Read the model definition and answer for the solid it produces. Units are mm, in the model's axes. Give positions to 0.01 mm unless a question says otherwise; leave off trailing zeros. Loops run counter-clockwise (first coordinate to the right, second up) from the corner with the lowest first, then second, coordinate; pieces in that order, holes last. Notation, with made-up numbers: (-27.75, 58) - (18.25, 58) arc R24 ccw to (18.25, 70) - close; hole circle Ø10 at (86, 20). An arc over 180 degrees is marked (long way). Put each result on its own line as item: value. Start each with the question number.
1. Given pin 1 Ø12 at (x, y) = (115.5, 28) entering from +Z; pin 2 Ø10 at (x, z) = (-159, 6.5) entering from +Y; pin 3 Ø6 at (x, y) = (-97, 34.5) entering from +Z; pin 4 Ø4.5 at (x, y) = (-194.5, -25) entering from -Z, each flat-ended and moving along its own axis, determine where each tip first touches the part or whether it passes through.
2. A cutting plane is placed at B-B, the plane y = 25.5. Determine the outline of the cut face in (x, z), plus the area to 3 significant figures.
3. Consider L1, parallel to Y at x = -422, z = 1.75; L2, parallel to Y at x = 131, z = 2.25; L3, parallel to Y at x = 32.5, z = 7.75. Determine where each line is inside the solid, lowest interval first. Write a range as from..to.
```python
from build123d import *

# Parameters (mm, degrees)
SKETCH1_W           = 1000
SKETCH1_H           = 100
BOSS_EXTRUDE1_DEPTH = 25
CUT_EXTRUDE1_DEPTH  = 1002.561281201
CUT_EXTRUDE2_DEPTH  = 1002.561281201
CUT_EXTRUDE3_DEPTH  = 1002.561281201
CUT_EXTRUDE4_DEPTH  = 1002.561281201
CUT_EXTRUDE5_DEPTH  = 10
CUT_EXTRUDE6_DEPTH  = 504.110335811
CUT_EXTRUDE7_DEPTH  = 10
CUT_EXTRUDE8_DEPTH  = 504.110335811
CUT_EXTRUDE9_DEPTH  = 10
CUT_EXTRUDE10_DEPTH = 504.110335811
CUT_EXTRUDE11_DEPTH = 10
CUT_EXTRUDE12_DEPTH = 504.110335811
CUT_EXTRUDE13_DEPTH = 10
CUT_EXTRUDE14_DEPTH = 504.110335811
CUT_EXTRUDE15_DEPTH = 10
CUT_EXTRUDE16_DEPTH = 504.110335811
CHAMFER1_SIZE       = 5.8
CHAMFER2_SIZE       = 1.5
FILLET1_R           = 1
FILLET2_R           = 3.2
FILLET3_R           = 6.3
CUT_EXTRUDE17_START = -250
CUT_EXTRUDE17_DEPTH = 250


with BuildPart() as part:
    # Sketch1 → Boss-Extrude1 (new body)
    with BuildSketch(Plane(origin=(0, 0, 0), x_dir=(-1, 0, 0), z_dir=(0, 0, -1))):
        Rectangle(SKETCH1_W, SKETCH1_H)
    extrude(amount=-BOSS_EXTRUDE1_DEPTH)

    # Sketch2 → Cut-Extrude1 (cut, through all)
    with BuildSketch(Plane(origin=(500, 0, 0), x_dir=(0, 0, -1), z_dir=(1, 0, 0))):
        Polygon((0, 37.3), (-15, 37.3), (-15, 12.7), (-0.1, 12.7), (-0.1, -12.7), (-15, -12.7), (-15, -37.3), (0, -37.3), align=None)
    extrude(amount=-CUT_EXTRUDE1_DEPTH, mode=Mode.SUBTRACT)

    # Sketch3 → Cut-Extrude2 (cut, through all)
    with BuildSketch(Plane(origin=(500, 0, 0), x_dir=(0, 0, -1), z_dir=(1, 0, 0))):
        with BuildLine():
            Line((-17.2, -50), (-5.7, -50))
            Line((-5.7, -50), (-5.7, -45.157716447))
            ThreePointArc((-5.7, -45.157716447), (-7.402384051, -42.609918665), (-10.407716447, -43.207716447))
            Line((-10.407716447, -43.207716447), (-17.2, -50))
        make_face()
    extrude(amount=-CUT_EXTRUDE2_DEPTH, mode=Mode.SUBTRACT)

    # Sketch4 → Cut-Extrude3 (cut, through all)
    with BuildSketch(Plane(origin=(500, 0, 0), x_dir=(0, 0, -1), z_dir=(1, 0, 0))):
        Polygon((-25, -42.243650814), (-20, -37.243650814), (-20, 37.243650814), (-25, 42.243650814), align=None)
    extrude(amount=-CUT_EXTRUDE3_DEPTH, mode=Mode.SUBTRACT)

    # Sketch5 → Cut-Extrude4 (cut, through all)
    with BuildSketch(Plane(origin=(500, 0, 0), x_dir=(0, 0, -1), z_dir=(1, 0, 0))):
        with BuildLine():
            Line((-5.7, 50), (-17.2, 50))
            Line((-17.2, 50), (-10.407716447, 43.207716447))
            ThreePointArc((-10.407716447, 43.207716447), (-7.402384051, 42.609918665), (-5.7, 45.157716447))
            Line((-5.7, 45.157716447), (-5.7, 50))
        make_face()
    extrude(amount=-CUT_EXTRUDE4_DEPTH, mode=Mode.SUBTRACT)

    # Sketch6 → Cut-Extrude5 (cut)
    with BuildSketch(Plane.XY.offset(20)):
        with BuildLine():
            Line((419.1, -5.5), (469.9, -5.5))
            ThreePointArc((469.9, -5.5), (475.4, 0), (469.9, 5.5))
            Line((469.9, 5.5), (419.1, 5.5))
            ThreePointArc((419.1, 5.5), (413.6, 0), (419.1, -5.5))
        make_face()
    extrude(amount=-CUT_EXTRUDE5_DEPTH, mode=Mode.SUBTRACT)

    # Sketch7 → Cut-Extrude6 (cut, through all)
    with BuildSketch(Plane(origin=(0, 0, 0.1), x_dir=(-1, 0, 0), z_dir=(0, 0, -1))):
        with BuildLine():
            Line((-469.9, -3.5), (-419.1, -3.5))
            ThreePointArc((-419.1, -3.5), (-415.6, 0), (-419.1, 3.5))
            Line((-419.1, 3.5), (-469.9, 3.5))
            ThreePointArc((-469.9, 3.5), (-473.4, 0), (-469.9, -3.5))
        make_face()
    extrude(amount=-CUT_EXTRUDE6_DEPTH, mode=Mode.SUBTRACT)

    # Sketch8 → Cut-Extrude7 (cut)
    with BuildSketch(Plane.XY.offset(20)):
        with BuildLine():
            Line((241.3, -5.5), (292.1, -5.5))
            ThreePointArc((292.1, -5.5), (297.6, 0), (292.1, 5.5))
            Line((292.1, 5.5), (241.3, 5.5))
            ThreePointArc((241.3, 5.5), (235.8, 0), (241.3, -5.5))
        make_face()
    extrude(amount=-CUT_EXTRUDE7_DEPTH, mode=Mode.SUBTRACT)

    # Sketch9 → Cut-Extrude8 (cut, through all)
    with BuildSketch(Plane(origin=(0, 0, 0.1), x_dir=(-1, 0, 0), z_dir=(0, 0, -1))):
        with BuildLine():
            Line((-292.1, -3.5), (-241.3, -3.5))
            ThreePointArc((-241.3, -3.5), (-237.8, 0), (-241.3, 3.5))
            Line((-241.3, 3.5), (-292.1, 3.5))
            ThreePointArc((-292.1, 3.5), (-295.6, 0), (-292.1, -3.5))
        make_face()
    extrude(amount=-CUT_EXTRUDE8_DEPTH, mode=Mode.SUBTRACT)

    # Sketch10 → Cut-Extrude9 (cut)
    with BuildSketch(Plane.XY.offset(20)):
        with BuildLine():
            Line((63.5, -5.5), (114.3, -5.5))
            ThreePointArc((114.3, -5.5), (119.8, 0), (114.3, 5.5))
            Line((114.3, 5.5), (63.5, 5.5))
            ThreePointArc((63.5, 5.5), (58, 0), (63.5, -5.5))
        make_face()
    extrude(amount=-CUT_EXTRUDE9_DEPTH, mode=Mode.SUBTRACT)

    # Sketch11 → Cut-Extrude10 (cut, through all)
    with BuildSketch(Plane(origin=(0, 0, 0.1), x_dir=(-1, 0, 0), z_dir=(0, 0, -1))):
        with BuildLine():
            Line((-114.3, -3.5), (-63.5, -3.5))
            ThreePointArc((-63.5, -3.5), (-60, 0), (-63.5, 3.5))
            Line((-63.5, 3.5), (-114.3, 3.5))
            ThreePointArc((-114.3, 3.5), (-117.8, 0), (-114.3, -3.5))
        make_face()
    extrude(amount=-CUT_EXTRUDE10_DEPTH, mode=Mode.SUBTRACT)

    # Sketch12 → Cut-Extrude11 (cut)
    with BuildSketch(Plane.XY.offset(20)):
        with BuildLine():
            Line((-114.3, -5.5), (-63.5, -5.5))
            ThreePointArc((-63.5, -5.5), (-58, 0), (-63.5, 5.5))
            Line((-63.5, 5.5), (-114.3, 5.5))
            ThreePointArc((-114.3, 5.5), (-119.8, 0), (-114.3, -5.5))
        make_face()
    extrude(amount=-CUT_EXTRUDE11_DEPTH, mode=Mode.SUBTRACT)

    # Sketch13 → Cut-Extrude12 (cut, through all)
    with BuildSketch(Plane(origin=(0, 0, 0.1), x_dir=(-1, 0, 0), z_dir=(0, 0, -1))):
        with BuildLine():
            Line((63.5, -3.5), (114.3, -3.5))
            ThreePointArc((114.3, -3.5), (117.8, 0), (114.3, 3.5))
            Line((114.3, 3.5), (63.5, 3.5))
            ThreePointArc((63.5, 3.5), (60, 0), (63.5, -3.5))
        make_face()
    extrude(amount=-CUT_EXTRUDE12_DEPTH, mode=Mode.SUBTRACT)

    # Sketch14 → Cut-Extrude13 (cut)
    with BuildSketch(Plane.XY.offset(20)):
        with BuildLine():
            Line((-292.1, -5.5), (-241.3, -5.5))
            ThreePointArc((-241.3, -5.5), (-235.8, 0), (-241.3, 5.5))
            Line((-241.3, 5.5), (-292.1, 5.5))
            ThreePointArc((-292.1, 5.5), (-297.6, 0), (-292.1, -5.5))
        make_face()
    extrude(amount=-CUT_EXTRUDE13_DEPTH, mode=Mode.SUBTRACT)

    # Sketch15 → Cut-Extrude14 (cut, through all)
    with BuildSketch(Plane(origin=(0, 0, 0.1), x_dir=(-1, 0, 0), z_dir=(0, 0, -1))):
        with BuildLine():
            Line((241.3, -3.5), (292.1, -3.5))
            ThreePointArc((292.1, -3.5), (295.6, 0), (292.1, 3.5))
            Line((292.1, 3.5), (241.3, 3.5))
            ThreePointArc((241.3, 3.5), (237.8, 0), (241.3, -3.5))
        make_face()
    extrude(amount=-CUT_EXTRUDE14_DEPTH, mode=Mode.SUBTRACT)

    # Sketch16 → Cut-Extrude15 (cut)
    with BuildSketch(Plane.XY.offset(20)):
        with BuildLine():
            Line((-469.9, -5.5), (-419.1, -5.5))
            ThreePointArc((-419.1, -5.5), (-413.6, 0), (-419.1, 5.5))
            Line((-419.1, 5.5), (-469.9, 5.5))
            ThreePointArc((-469.9, 5.5), (-475.4, 0), (-469.9, -5.5))
        make_face()
    extrude(amount=-CUT_EXTRUDE15_DEPTH, mode=Mode.SUBTRACT)

    # Sketch17 → Cut-Extrude16 (cut, through all)
    with BuildSketch(Plane(origin=(0, 0, 0.1), x_dir=(-1, 0, 0), z_dir=(0, 0, -1))):
        with BuildLine():
            Line((419.1, -3.5), (469.9, -3.5))
            ThreePointArc((469.9, -3.5), (473.4, 0), (469.9, 3.5))
            Line((469.9, 3.5), (419.1, 3.5))
            ThreePointArc((419.1, 3.5), (415.6, 0), (419.1, -3.5))
        make_face()
    extrude(amount=-CUT_EXTRUDE16_DEPTH, mode=Mode.SUBTRACT)

    # Chamfer1
    chamfer1_edges = [part.edges().sort_by_distance(p)[0] for p in [
        (0, -12.7, 15),
        (0, 12.7, 15),
    ]]
    chamfer(chamfer1_edges, length=CHAMFER1_SIZE)

    # Chamfer2
    chamfer2_edges = [part.edges().sort_by_distance(p)[0] for p in [
        (500, -50, 2.85),
        (-500, -50, 2.85),
        (-500, 50, 21.1),
        (-500, -50, 21.1),
        (500, -50, 21.1),
        (500, 50, 2.85),
        (500, 50, 21.1),
        (-500, 50, 2.85),
    ]]
    chamfer(chamfer2_edges, length=CHAMFER2_SIZE)

    # Fillet1
    fillet1_edges = [part.edges().sort_by_distance(p)[0] for p in [
        (0, 50, 25),
        (0, -50, 25),
    ]]
    fillet(fillet1_edges, radius=FILLET1_R)

    # Fillet2
    fillet2_edges = [part.edges().sort_by_distance(p)[0] for p in [
        (0, -37.3, 15),
        (0, 37.3, 15),
    ]]
    fillet(fillet2_edges, radius=FILLET2_R)

    # Fillet3
    fillet3_edges = [part.edges().sort_by_distance(p)[0] for p in [
        (0, 37.243650814, 20),
        (0, -37.243650814, 20),
    ]]
    fillet(fillet3_edges, radius=FILLET3_R)

    # Sketch18 → Cut-Extrude17 (cut)
    with BuildSketch(Plane(origin=(500, 0, 0), x_dir=(0, 0, -1), z_dir=(1, 0, 0)).offset(CUT_EXTRUDE17_START)):
        with BuildLine():
            Line((-5.7, 50), (-5.7, 48.5))
            Line((-5.7, 48.5), (-5.7, 45.157716447))
            ThreePointArc((-5.7, 45.157716447), (-7.402384051, 42.609918665), (-10.407716447, 43.207716447))
            Line((-10.407716447, 43.207716447), (-15.7, 48.5))
            Line((-15.7, 48.5), (-17.2, 50))
            Line((-17.2, 50), (-24, 50))
            ThreePointArc((-24, 50), (-24.707106781, 49.707106781), (-25, 49))
            Line((-25, 49), (-25, 48.5))
            Line((-25, 48.5), (-25, 42.243650814))
            Line((-25, 42.243650814), (-21.845227279, 39.088878092))
            ThreePointArc((-21.845227279, 39.088878092), (-20.479558945, 37.045010995), (-20, 34.634105371))
            Line((-20, 34.634105371), (-20, -34.634105371))
            ThreePointArc((-20, -34.634105371), (-20.479558945, -37.045010995), (-21.845227279, -39.088878092))
            Line((-21.845227279, -39.088878092), (-25, -42.243650814))
            Line((-25, -42.243650814), (-25, -48.5))
            Line((-25, -48.5), (-25, -49))
            ThreePointArc((-25, -49), (-24.707106781, -49.707106781), (-24, -50))
            Line((-24, -50), (-17.2, -50))
            Line((-17.2, -50), (-15.7, -48.5))
            Line((-15.7, -48.5), (-10.407716447, -43.207716447))
            ThreePointArc((-10.407716447, -43.207716447), (-7.402384051, -42.609918665), (-5.7, -45.157716447))
            Line((-5.7, -45.157716447), (-5.7, -48.5))
            Line((-5.7, -48.5), (-5.7, -50))
            Line((-5.7, -50), (0, -50))
            Line((0, -50), (0, -48.5))
            Line((0, -48.5), (0, -37.3))
            Line((0, -37.3), (-11.8, -37.3))
            ThreePointArc((-11.8, -37.3), (-14.0627417, -36.3627417), (-15, -34.1))
            Line((-15, -34.1), (-15, -18.5))
            Line((-15, -18.5), (-9.2, -12.7))
            Line((-9.2, -12.7), (-0.1, -12.7))
            Line((-0.1, -12.7), (-0.1, 12.7))
            Line((-0.1, 12.7), (-9.2, 12.7))
            Line((-9.2, 12.7), (-15, 18.5))
            Line((-15, 18.5), (-15, 34.1))
            ThreePointArc((-15, 34.1), (-14.0627417, 36.3627417), (-11.8, 37.3))
            Line((-11.8, 37.3), (0, 37.3))
            Line((0, 37.3), (0, 48.5))
            Line((0, 48.5), (0, 50))
            Line((0, 50), (-5.7, 50))
        make_face()
    extrude(amount=CUT_EXTRUDE17_DEPTH, mode=Mode.SUBTRACT)


solid = part.part
```
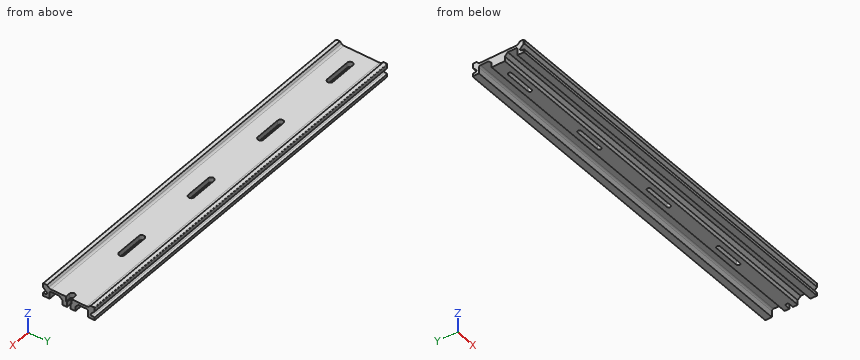
Return value:
1. pin 1: stops at z = 20
1. pin 2: stops at y = 50
1. pin 3: stops at z = 20.69
1. pin 4: stops at z = 15
2. outline: (-500, 15) - (250, 15) - (250, 20) - (-500, 20) - close
2. area: 3,750 mm2
3. L1: y = -50..-37.3, -12.7..-3.5, 3.5..12.7, 37.3..50
3. L2: y = -50..-37.3, -12.7..12.7, 37.3..50
3. L3: y = -42.49..-37.3, -12.7..12.7, 37.3..42.49
